The model under review builds one solid part; all positions refer to its coordinate system, in mm. Round coordinates to 2 decimals unless told otherwise and drop trailing zeros. Loops run counter-clockwise (first coordinate to the right, second up) from the corner with the lowest first, then second, coordinate; pieces in that order, holes last. Notation, with made-up numbers: M 67,67.5 L 76,67.5 A22 cw 76,73.5 Z; hole C 12,58 d10. An arc over 180 degrees is marked long. Return JSON: item names as keys, results as strings. Group by question number.
Q1. Consider section A-A (y = -25). State the section outline as (x, z) points, and give its area (3 significant figures).
Q2. To check wall thickness, follow line 1 along X through (y, z) = (-1.1, 0); line 2 along X through (y, z) = (-13.5, 12); line 3 along Z through (x, y) = (270.5, -26). State the ranges of each line that lie inside material, in increasing order.
Q3. Clearance check with flat-ended pins moving along their axes: pin 1 Ø4 at (y, z) = (-8.5, 259.5) entering from -X; pin 2 Ø12 at (y, z) = (-19, -184) entering from -X; pin 3 Ø11.5 at (x, z) = (276.83, -276.83) entering from -Y. State where each tip first meets the part, or that it passes through.
from build123d import *

# Parameters (mm, degrees)
SKETCH1_R          = 406.5
SKETCH1_R_2        = 376.5
BASE_FLANGE1_DEPTH = 2.5
SKETCH8_R          = 5
CUT_EXTRUDE1_DEPTH = 10


# Read off the part's stored shape, not the designer's step: Edge-Flange1
# Sheet-metal steps are written as plain solids
with BuildPart() as part:
    # Sketch1 → Base-Flange1 (new body)
    with BuildSketch(Plane(origin=(0, 0, 0), x_dir=(1, 0, 0), z_dir=(0, 1, 0))):
        with Locations(Location((0, 0, 0), (0, 0, 270))):
            Circle(SKETCH1_R)
        with Locations(Location((0, 0, 0), (0, 0, 270))):
            Circle(SKETCH1_R_2, mode=Mode.SUBTRACT)
    extrude(amount=-BASE_FLANGE1_DEPTH)

    # Edge-Flange1 outline → Edge-Flange1 (revolve, cut)
    with BuildSketch(Plane.XY):
        with BuildLine():
            Line((376.5, -2.5), (376.645898034, -2.5))
            ThreePointArc((376.645898034, -2.5), (377.908349934, -0.69375696), (380, 0))
            Line((380, 0), (376.5, 0))
            Line((376.5, 0), (376.5, -2.5))
        make_face()
    revolve(axis=Axis((0, 0, 0), (0, 1, 0)), mode=Mode.SUBTRACT)

    # Edge-Flange1 2 outline → Edge-Flange1 2 (revolve)
    with BuildSketch(Plane.XY):
        with BuildLine():
            Line((376.5, -3.5), (376.5, -32.5))
            Line((376.5, -32.5), (379, -32.5))
            Line((379, -32.5), (379, -3.5))
            ThreePointArc((379, -3.5), (379.292893219, -2.792893219), (380, -2.5))
            Line((380, -2.5), (376.645898034, -2.5))
            ThreePointArc((376.645898034, -2.5), (376.536666571, -2.994706462), (376.5, -3.5))
        make_face()
    revolve(axis=Axis((0, 0, 0), (0, 1, 0)))

    # Sketch8 → Cut-Extrude1 (cut)
    with BuildSketch(Plane(origin=(0, 0, 0), x_dir=(1, 0, 0), z_dir=(0, 1, 0))):
        with Locations(Location((149.820563771, 361.698836978, 0), (0, 0, 270))):
            Circle(SKETCH8_R)
        with Locations(Location((276.832304835, 276.832304835, 0), (0, 0, 270))):
            Circle(SKETCH8_R)
        with Locations(Location((0, 391.5, 0), (0, 0, 270))):
            Circle(SKETCH8_R)
        with Locations(Location((361.698836978, 149.820563771, 0), (0, 0, 270))):
            Circle(SKETCH8_R)
        with Locations(Location((391.5, 0, 0), (0, 0, 270))):
            Circle(SKETCH8_R)
        with Locations(Location((361.698836978, -149.820563771, 0), (0, 0, 270))):
            Circle(SKETCH8_R)
        with Locations(Location((276.832304835, -276.832304835, 0), (0, 0, 270))):
            Circle(SKETCH8_R)
        with Locations(Location((149.820563771, -361.698836978, 0), (0, 0, 270))):
            Circle(SKETCH8_R)
        with Locations(Location((0, -391.5, 0), (0, 0, 270))):
            Circle(SKETCH8_R)
        with Locations(Location((-149.820563771, -361.698836978, 0), (0, 0, 270))):
            Circle(SKETCH8_R)
        with Locations(Location((-276.832304834, -276.832304835, 0), (0, 0, 270))):
            Circle(SKETCH8_R)
        with Locations(Location((-361.698836978, -149.820563771, 0), (0, 0, 270))):
            Circle(SKETCH8_R)
        with Locations(Location((-391.5, 0, 0), (0, 0, 270))):
            Circle(SKETCH8_R)
        with Locations(Location((-361.698836978, 149.820563771, 0), (0, 0, 270))):
            Circle(SKETCH8_R)
        with Locations(Location((-276.832304835, 276.832304835, 0), (0, 0, 270))):
            Circle(SKETCH8_R)
        with Locations(Location((-149.820563771, 361.698836978, 0), (0, 0, 270))):
            Circle(SKETCH8_R)
    extrude(amount=-CUT_EXTRUDE1_DEPTH, mode=Mode.SUBTRACT)


solid = part.part
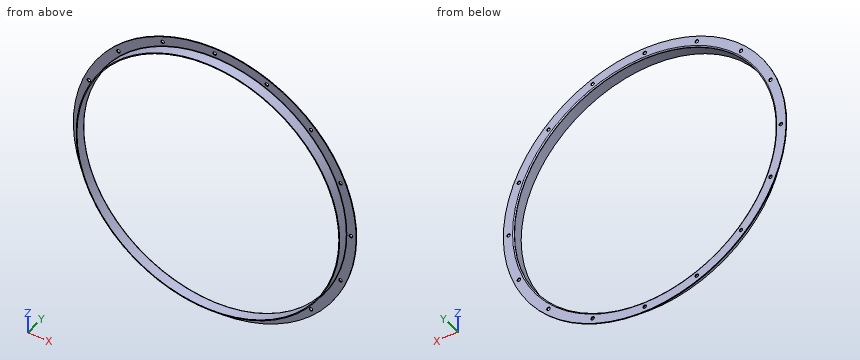
Values:
{
 "1": {"outline": "C 0,0 d758; hole C 0,0 d753", "area": "5,930 mm2"},
 "2": {"line 1": "x = -406.5 to -396.5, -386.5 to -377.45, 377.45 to 386.5, 396.5 to 406.5", "line 2": "x = -378.81 to -376.31, 376.31 to 378.81", "line 3": "z = -265.46 to -261.88, 261.88 to 265.46"},
 "3": {"pin 1": "stops at x = -278.09", "pin 2": "stops at x = -334.6", "pin 3": "stops at y = -2.5"}
}
